Build history of the part. All positions in model axes, mm. Face numbers are marked on the shaded views. A direction names the side the tool comes from. Round coordinates to 2 decimals unless told otherwise and drop trailing zeros. Order: outer loops, then holes, each group sorted by start corner. A loop starts at its lowest first (then second) coordinate and runs counter-clockwise, first axis right, second up. Notation, with made-up numbers: M -22.5,68 L 31.5,68 A16 cw 31.5,96 Z; hole C 46.25,-28.75 d1. An arc over 180 degrees is marked long. One line per item, written item: value. Start each with the question number.
Item 1: Two-plate mould, pull along X, no slides. Class the marked faces 5, 6 and 7: +X half, -X half, draft (parallel to the pull), parting line (faces both ways), or undercut.
Item 2: Pin check, flat tips, straight feed: pin 1 (1.5 mm diameter, centred on x = 134.5, z = -31, fed in from +Y); pin 2 (23 mm diameter, centred on y = 69, z = -7.5, fed in from +X); pin 3 (16 mm diameter, centred on y = 98, z = 20, fed in from +X); pin 4 (6 mm diameter, centred on y = 93.5, z = 27, fed in from +X). Stop position of each tip, or through.
Item 3: Band-saw the part on A-A, the plane y = 11.5. Write the cut outline in (x, z).
Item 4: Band-saw the part on B-B, the plane z = -46. Write the cut outline in (x, y).
Item 5: Probe L1, parallel to X at y = 88, z = -33; L2, parallel to X at y = 40, z = 58; L3, parallel to X at y = 23.5, z = -1. List the from-to ranges inside material, lowest first.
Item 6: Tool access for the marked faces 1, 2, 3 and 4: list every direction of +Z, -Z, +X, -X, +Y, -Y with a clear straight run to the whole face (end or side of a thin tool).
Item 7: Band-saw the part on C-C, the plane z = 3. Write the cut outline in (x, y), then the cut area to 3 significant figures.
Item 8: Band-saw the part on D-D, the plane x = -53. Write the cut outline in (y, z).
```python
from build123d import *

# Parameters (mm, degrees)
SKETCH1_W           = 150
SKETCH1_H           = 84
SKETCH1_R           = 12
BOSS_EXTRUDE1_DEPTH = 16
SKETCH4_W           = 16
SKETCH4_H           = 84
BOSS_EXTRUDE2_DEPTH = 28
SKETCH5_W           = 84
SKETCH5_H           = 16
BOSS_EXTRUDE3_DEPTH = 98
SKETCH7_W           = 60
SKETCH7_H           = 16
BOSS_EXTRUDE4_DEPTH = 46
FILLET2_R           = 30
FILLET3_R           = 16
CUT_EXTRUDE1_REACH  = 201.02
SKETCH9_R           = 12
SKETCH11_R          = 10
BOSS_EXTRUDE5_DEPTH = 16
SKETCH13_W          = 16
SKETCH13_H          = 42
BOSS_EXTRUDE6_DEPTH = 104
FILLET4_R           = 22
CUT_EXTRUDE2_REACH  = 291.22
SKETCH15_R          = 10
SKETCH14_W          = 16
SKETCH14_H          = 44
BOSS_EXTRUDE8_DEPTH = 72
CUT_EXTRUDE3_REACH  = 291.22
SKETCH16_R          = 10
FILLET5_R           = 22


with BuildPart() as part:
    # Sketch1 → Boss-Extrude1 (new body)
    with BuildSketch(Plane(origin=(0, 0, 0), x_dir=(1, 0, 0), z_dir=(0, 1, 0))):
        Rectangle(SKETCH1_W, SKETCH1_H)
        with Locations(Location((0, 0, 0), (0, 0, 270))):
            Circle(SKETCH1_R, mode=Mode.SUBTRACT)
    extrude(amount=BOSS_EXTRUDE1_DEPTH)

    # Sketch4 → Boss-Extrude2 (add)
    with BuildSketch(Plane(origin=(0, 16, 0), x_dir=(1, 0, 0), z_dir=(0, 1, 0))):
        with Locations((67, 0)):
            Rectangle(SKETCH4_W, SKETCH4_H)
    extrude(amount=BOSS_EXTRUDE2_DEPTH)

    # Sketch5 → Boss-Extrude3 (add)
    with BuildSketch(Plane(origin=(75, 0, 0), x_dir=(0, 0, -1), z_dir=(1, 0, 0))):
        with Locations((0, 36)):
            Rectangle(SKETCH5_W, SKETCH5_H)
    extrude(amount=BOSS_EXTRUDE3_DEPTH)

    # Sketch7 → Boss-Extrude4 (add)
    with BuildSketch(Plane.XY.offset(42)):
        with Locations((143, 36)):
            Rectangle(SKETCH7_W, SKETCH7_H)
    extrude(amount=BOSS_EXTRUDE4_DEPTH)

    # Fillet2
    fillet2_edges = [part.edges().sort_by_distance(p)[0] for p in [
        (173, 36, 88),
        (173, 36, -42),
        (113, 36, 88),
    ]]
    fillet(fillet2_edges, radius=FILLET2_R - 0.0001)  # a hair under: the kernel refuses the full size

    # Fillet3
    fillet3_edges = [part.edges().sort_by_distance(p)[0] for p in [
        (113, 36, 42),
    ]]
    fillet(fillet3_edges, radius=FILLET3_R)

    # Sketch9 → Cut-Extrude1 (cut, up to next)
    with BuildSketch(Plane(origin=(0, 44, 0), x_dir=(1, 0, 0), z_dir=(0, 1, 0)), mode=Mode.PRIVATE) as cut_extrude1_sk1:
        with Locations(Location((143, 12, 0), (0, 0, 270))):
            Circle(SKETCH9_R)
    cut_extrude1_tool1 = extrude(cut_extrude1_sk1.sketch, amount=-CUT_EXTRUDE1_REACH, mode=Mode.PRIVATE) & part.part
    # Sketch9 → Cut-Extrude1 (cut, up to next)
    with BuildSketch(Plane(origin=(0, 44, 0), x_dir=(1, 0, 0), z_dir=(0, 1, 0)), mode=Mode.PRIVATE) as cut_extrude1_sk2:
        with Locations(Location((143, -58, 0), (0, 0, 270))):
            Circle(SKETCH9_R)
    cut_extrude1_tool2 = extrude(cut_extrude1_sk2.sketch, amount=-CUT_EXTRUDE1_REACH, mode=Mode.PRIVATE) & part.part
    add(cut_extrude1_tool1.solids().sort_by_distance((143, 44, -12))[0], mode=Mode.SUBTRACT)
    add(cut_extrude1_tool2.solids().sort_by_distance((143, 44, 58))[0], mode=Mode.SUBTRACT)

    # Sketch11 → Boss-Extrude5 (add)
    with BuildSketch(Plane.ZY.offset(-59)):
        with BuildLine():
            Line((-42, 44), (-68.617604355, 86.278873429))
            ThreePointArc((-68.617604355, 86.278873429), (-64.123788111, 114.867679431), (-35.190151029, 114.268631579))
            Line((-35.190151029, 114.268631579), (42, 44))
            Line((42, 44), (-42, 44))
        make_face()
        with Locations((-50, 98)):
            Circle(SKETCH11_R, mode=Mode.SUBTRACT)
    extrude(amount=-BOSS_EXTRUDE5_DEPTH)

    # Sketch13 → Boss-Extrude6 (add)
    with BuildSketch(Plane(origin=(0, 16, 0), x_dir=(1, 0, 0), z_dir=(0, 1, 0))):
        with Locations((-67, -21)):
            Rectangle(SKETCH13_W, SKETCH13_H)
    extrude(amount=BOSS_EXTRUDE6_DEPTH)

    # Fillet4
    fillet4_edges = [part.edges().sort_by_distance(p)[0] for p in [
        (-67, 120, 42),
    ]]
    fillet(fillet4_edges, radius=FILLET4_R)

    # Sketch15 → Cut-Extrude2 (cut, up to next)
    with BuildSketch(Plane.ZY.offset(75), mode=Mode.PRIVATE) as cut_extrude2_sk1:
        with Locations((20, 98)):
            Circle(SKETCH15_R)
    cut_extrude2_tool1 = extrude(cut_extrude2_sk1.sketch, amount=-CUT_EXTRUDE2_REACH, mode=Mode.PRIVATE) & part.part
    add(cut_extrude2_tool1.solids().sort_by_distance((-75, 98, 20))[0], mode=Mode.SUBTRACT)

    # Sketch14 → Boss-Extrude8 (add)
    with BuildSketch(Plane(origin=(0, 0, 0), x_dir=(-1, 0, 0), z_dir=(0, 0, -1))):
        with Locations((67, 98)):
            Rectangle(SKETCH14_W, SKETCH14_H)
    extrude(amount=BOSS_EXTRUDE8_DEPTH)

    # Sketch16 → Cut-Extrude3 (cut, up to next)
    with BuildSketch(Plane.ZY.offset(75), mode=Mode.PRIVATE) as cut_extrude3_sk1:
        with Locations((-50, 98)):
            Circle(SKETCH16_R)
    cut_extrude3_tool1 = extrude(cut_extrude3_sk1.sketch, amount=-CUT_EXTRUDE3_REACH, mode=Mode.PRIVATE) & part.part
    add(cut_extrude3_tool1.solids().sort_by_distance((-75, 98, -50))[0], mode=Mode.SUBTRACT)

    # Fillet5
    fillet5_edges = [part.edges().sort_by_distance(p)[0] for p in [
        (-67, 120, -72),
        (-67, 76, -72),
    ]]
    fillet(fillet5_edges, radius=FILLET5_R - 0.0001)  # a hair under: the kernel refuses the full size


solid = part.part
```
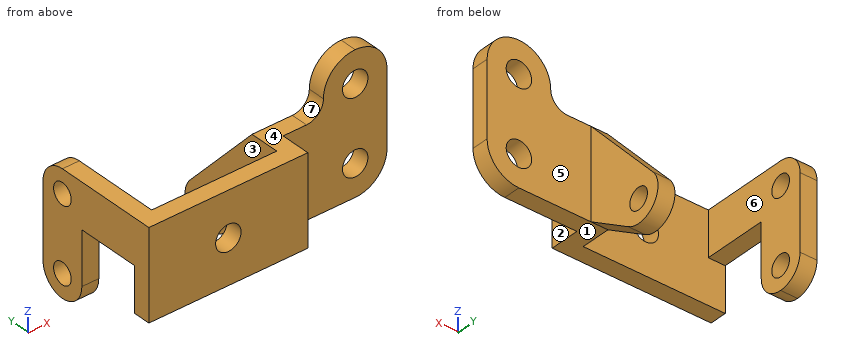
Output:
1. face 5: draft
1. face 6: undercut
1. face 7: -X half
2. pin 1: stops at y = 44
2. pin 2: stops at x = 75
2. pin 3: passes through
2. pin 4: stops at x = -59
3. outline: M -75,-42 L 75,-42 L 75,42 L -75,42 Z; hole C 0,0 d24
4. outline: M -75,76 L -59,76 L -59,88.83 L -75,88.83 Z; M -75,107.17 L -59,107.17 L -59,120 L -75,120 Z; M 59,50.35 L 75,50.35 L 75,88.83 L 59,88.83 Z; M 59,107.17 L 75,107.17 L 75,119.63 L 59,119.63 Z
5. L1: x = -75 to -59, 59 to 75
5. L2: x = 113 to 131, 155 to 173
5. L3: x = 59 to 75
6. face 1: -Z, +X, -X, -Y
6. face 2: +Z, -Z, +X, -Y
6. face 3: +Z, -Z, +Y
6. face 4: +Z, -X, +Y, -Y
7. outline: M -75,0 L -11.62,0 L -11.62,16 L -59,16 L -59,120 L -75,120 Z; M 11.62,0 L 75,0 L 75,28 L 173,28 L 173,44 L 75,44 L 75,79.5 L 59,79.5 L 59,16 L 11.62,16 Z
7. area: 6,280 mm²
8. outline: M 0,-42 L 16,-42 L 16,42 L 0,42 Z
